For this review, take the finished solid that the model builds, in its own axes (mm). A direction names the side the tool comes from. Give positions to 0.01 mm unless a question says otherwise; leave off trailing zeros. Order: outer loops, then holes, each group sorted by start corner. A loop starts at its lowest first (then second) coordinate and runs counter-clockwise, first axis right, second up. Notation, with made-up numbers: M -13,-4 L -4,-4 A26 cw -4,25 Z; hole C 81.5,44 d8. An arc over 180 degrees is marked long. Use CSV: the item, a comma, the result in double quotes. Start each with the question number.
(1) Consider section D-D (x = 346). Write out the cut boundary in (y, z), and give its area (3 significant figures).
(2) Draft analysis for pull direction Y (two halves, no side actions). For faces 1 (the face through (-315, -1300, 9)), 2 (the face through (-311.98, -1183.2, 5.44)), 3 (the face through (-315, -2200, 9)), state which applies: pulls with the +Y half, pulls with the -Y half, needs draft (parallel to the pull), parting line crosses it, or undercut.
(3) Consider section C-C (z = 70.5). Write out the cut boundary in (x, y), and give its area (3 significant figures).
(4) Clearance check with flat-ended pins moving along their axes: P1, Ø5, axis at x = 325, y = -1924, coming from the -Z side; P2, Ø3, axis at y = -1408, z = -20, coming from the -X side; P3, Ø10, axis at x = 356, y = -351, coming from the +Z side. State where each tip first meets the part, or that it passes through.
(5) Tool access review of faces 4 (the face through (-315.411, -1183.2, 9.105)), 5 (the face through (32, -1183, -151.535)): name each direction out of +Z, -Z, +X, -X, +Y, -Y from which nothing blocks a thin tool from reaching the whole face with its end or side.
(6) Consider section A-A (y = -301.5). Write out the cut boundary in (x, z), and give its area (3 significant figures).
(7) Consider section B-B (x = -301.5). Write out the cut boundary in (y, z), and give its area (3 significant figures).
(8) Wall thickness on L1, parallel to Z at x = -118, y = -1349; L2, parallel to X at y = -1985.5, z = -104.5; L3, parallel to X at y = -299.5, z = 87: over which ranges is each line inside the solid? List them lowest first. Write a range as from..to.
```python
from build123d import *

# Parameters (mm, degrees)
F1_DEPTH = 2400
F2_W     = 900
F2_H     = 250
F3_DEPTH = 1.6
F4_W     = 900
F4_H     = 250
F5_DEPTH = 1.6


with BuildPart() as f1:
    # F0 (on Front) → F1 (new body)
    with BuildSketch(Plane.XZ):
        Polygon((-239.018946, -140.479133), (-388.218946, 157.920867), (-392.691082, 166.865139), (-394.291082, 166.865139), (-234.291082, -153.134861), (290.052568, -153.134861), (450.052568, 166.865139), (448.452568, 166.865139), (443.980432, 157.920867), (294.780432, -140.479133), (289.252568, -151.534861), (276.891889, -151.534861), (-221.130403, -151.534861), (-233.491082, -151.534861), align=None)
    extrude(amount=F1_DEPTH)

    # F2 (on face) → F3 (cut)
    with BuildSketch(Plane(origin=(-248.68681, 0, -124.343405), x_dir=(0, -1, 0), z_dir=(-0.894427, 0, -0.447214))):
        with Locations((1750, 150.58105)):
            Rectangle(F2_W, F2_H)
    extrude(amount=-F3_DEPTH, mode=Mode.SUBTRACT)

    # F4 (on face) → F5 (cut)
    with BuildSketch(Plane(origin=(-248.68681, 0, -124.343405), x_dir=(0, -1, 0), z_dir=(-0.894427, 0, -0.447214))):
        with Locations((650, 150.58105)):
            Rectangle(F4_W, F4_H)
    extrude(amount=-F5_DEPTH, mode=Mode.SUBTRACT)


solid = f1.part
```
Check result:
1,outline,"M -2400,-41.24 L 0,-41.24 L 0,-38.04 L -2400,-38.04 Z"
1,area,"7,680 mm^2"
2,face 1,"undercut"
2,face 2,"needs draft"
2,face 3,"undercut"
3,outline,"M -346.11,-2400 L -344.51,-2400 L -344.51,-2200 L -346.11,-2200 Z; M -346.11,-1300 L -344.51,-1300 L -344.51,-1100 L -346.11,-1100 Z; M -346.11,-200 L -344.51,-200 L -344.51,0 L -346.11,0 Z; M 400.27,-2400 L 401.87,-2400 L 401.87,0 L 400.27,0 Z"
3,area,"4,800 mm^2"
4,P1,"stops at z = -88.24"
4,P2,"stops at x = 354.27"
4,P3,"stops at z = -8.04"
5,face 4,"-Z, -X, +Y, -Y"
5,face 5,"+Z, +Y, -Y"
6,outline,"M -394.29,166.87 L -371.93,122.14 L -370.65,122.78 L -392.69,166.87 Z; M -260.13,-101.46 L -234.29,-153.13 L 290.05,-153.13 L 450.05,166.87 L 448.45,166.87 L 289.25,-151.53 L -233.49,-151.53 L -258.85,-100.82 Z"
6,area,"1,500 mm^2"
7,outline,"M -2400,-18.72 L -2200,-18.72 L -2200,-15.52 L -2400,-15.52 Z; M -1300,-18.72 L -1100,-18.72 L -1100,-15.52 L -1300,-15.52 Z; M -200,-18.72 L 0,-18.72 L 0,-15.52 L -200,-15.52 Z"
7,area,"1,920 mm^2"
8,L1,"z = -153.13..-151.53"
8,L2,"x = -258.61..-257.01, 312.77..314.37"
8,L3,"x = 408.52..410.12"
